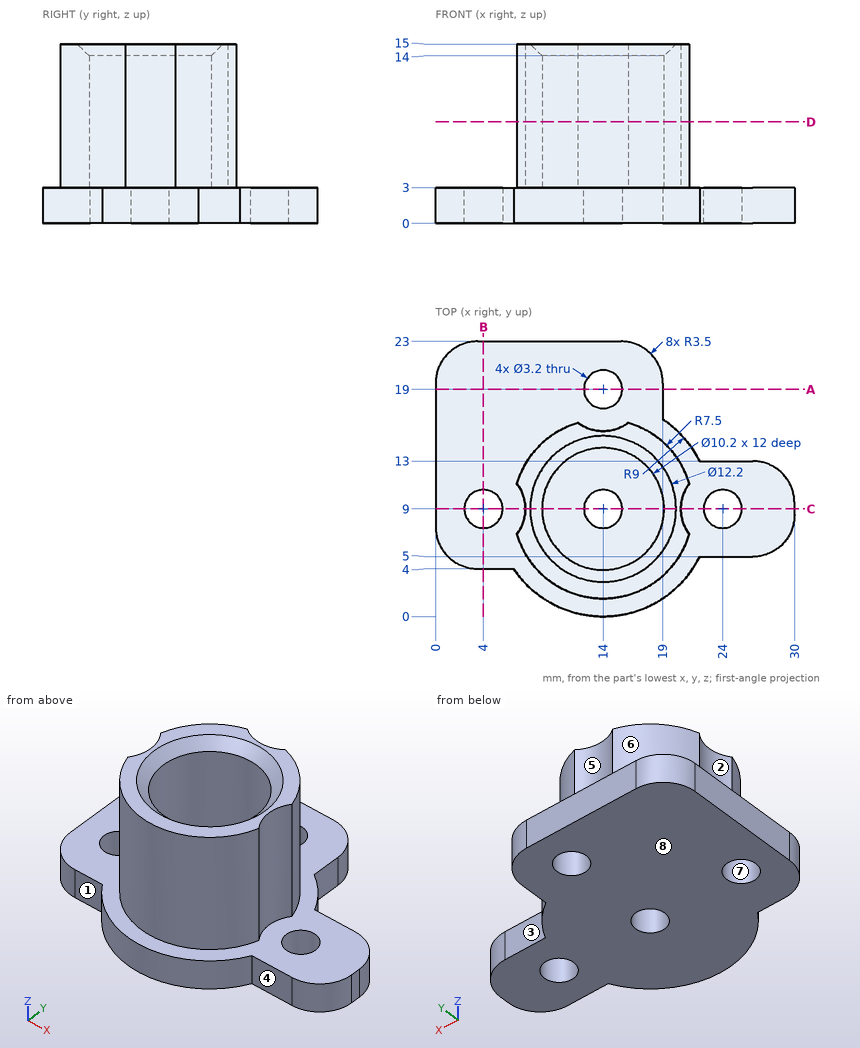
Study the drawing (mm; zero at the part's minimum x, y, z) and answer. A direction names the side the tool comes from. Give positions to 0.01 mm unless a question says otherwise; leave off trailing zeros. Write each loop counter-clockwise with the first axis right and the second up, starting at its lowest first coordinate (ties: lowest second). Pieces come first, ordered by that corner, then holes.
Item 1: Section A-A, the plane y = 19 is taken. Write down the section's boundary in (x, z), plus the area to 3 significant figures.
Item 2: Section D-D, the plane z = 8.5 is taken. Write down the section's boundary in (x, y), plus the area to 3 significant figures.
Item 3: Flat-ended cylindrical pins translate along their axes: P1, Ø11.5, axis at x = 14, y = 9, coming from the +Z side; P2, Ø5, axis at x = 14, y = 9, coming from the +Z side; P3, Ø1, axis at y = 13.5, z = 8, coming from the +X side. Find the tip coordinate at first contact, or state that the pin passes through.
Item 4: Find the intervals of material crossed by line 1 along Y through (x, z) = (14, 1.55); line 2 along Y through (x, z) = (4, 0.75); line 3 along Z through (x, y) = (9.5, 15.5), in increasing order.
Item 5: Determine the mould class of the marked faces 6, 7 and 8 for opening direction Y: released by +Y, released by -Y, zero draft, split by the parting line, or undercut.
Item 6: Which of the six approach directions +Z, -Z, +X, -X, +Y, -Y give full straight-line access (tool end or side, diameter ignored) to the marked faces 1, 2, 3, 4 and 5?
Item 7: Section B-B, the plane x = 4 is taken. Write down the section's boundary in (y, z), plus the area to 3 significant figures.
Item 8: Section C-C, the plane y = 9 is taken. Write down the section's boundary in (x, z), plus the area to 3 significant figures.
Completed:
1. outline: (0, 0) - (12.4, 0) - (12.4, 3) - (0, 3) - close; (15.6, 0) - (19, 0) - (19, 3) - (15.6, 3) - close
1. area: 47.4 mm2
2. outline: (6.8, 6.9) arc R7.5 ccw to (21.2, 6.9) arc R3.5 cw to (21.2, 11.1) arc R7.5 ccw to (16.1, 16.2) arc R3.5 cw to (11.9, 16.2) arc R7.5 ccw to (6.8, 11.1) arc R3.5 cw to start; hole circle Ø10.2 at (14, 9)
2. area: 86.5 mm2
3. P1: stops at z = 14.65
3. P2: stops at z = 3
3. P3: stops at x = 20.34
4. line 1: y = 0 to 7.4, 10.6 to 17.4, 20.6 to 23
4. line 2: y = 4 to 7.4, 10.6 to 23
4. line 3: z = 0 to 3
5. face 6: released by +Y
5. face 7: undercut
5. face 8: zero draft
6. face 1: +Z, -Z, -X, -Y
6. face 2: +Z, -X
6. face 3: +Z, -Z, +X, +Y
6. face 4: +Z, -Z, +X, -Y
6. face 5: +Z, +Y
7. outline: (4, 0) - (7.4, 0) - (7.4, 3) - (4, 3) - close; (10.6, 0) - (23, 0) - (23, 3) - (10.6, 3) - close
7. area: 47.4 mm2
8. outline: (0, 0) - (2.4, 0) - (2.4, 3) - (0, 3) - close; (5.6, 0) - (12.4, 0) - (12.4, 3) - (8.9, 3) - (8.9, 14) - (7.9, 15) - (7.5, 15) - (7.5, 3) - (5.6, 3) - close; (15.6, 0) - (22.4, 0) - (22.4, 3) - (20.5, 3) - (20.5, 15) - (20.1, 15) - (19.1, 14) - (19.1, 3) - (15.6, 3) - close; (25.6, 0) - (30, 0) - (30, 3) - (25.6, 3) - close
8. area: 93.8 mm2
